from build123d import *

# Parameters (mm, degrees)
ESBO_O1_R                = 12
RESSALTO_EXTRUS_O1_DEPTH = 9.6
ESBO_O2_R                = 11.4
CORTE_EXTRUS_O1_DEPTH    = 0.1
ESBO_O3_R                = 0.5
RESSALTO_EXTRUS_O2_DEPTH = 2
ESBO_O4_R                = 1.2
CORTE_EXTRUS_O2_DEPTH    = 2
ESBO_O5_R                = 3
CORTE_EXTRUS_O3_DEPTH    = 0.3
FILETE1_R                = 1


with BuildPart() as part:
    # Esboço1 → Ressalto-extrusão1 (new body)
    with BuildSketch(Plane.XY):
        Circle(ESBO_O1_R)
    extrude(amount=RESSALTO_EXTRUS_O1_DEPTH)

    # Esboço2 → Corte-extrusão1 (cut)
    with BuildSketch(Plane(origin=(0, 0, 0), x_dir=(-1, 0, 0), z_dir=(0, 0, -1))):
        Circle(ESBO_O2_R)
    extrude(amount=-CORTE_EXTRUS_O1_DEPTH, mode=Mode.SUBTRACT)

    # Esboço3 → Ressalto-extrusão2 (add)
    with BuildSketch(Plane(origin=(0, 0, 0.1), x_dir=(-1, 0, 0), z_dir=(0, 0, -1))):
        with Locations((6, 0)):
            Circle(ESBO_O3_R)
        with Locations((-6, 0)):
            Circle(ESBO_O3_R)
    extrude(amount=RESSALTO_EXTRUS_O2_DEPTH)

    # Esboço4 → Corte-extrusão2 (cut)
    with BuildSketch(Plane.XY.offset(9.6)):
        Circle(ESBO_O4_R)
    extrude(amount=-CORTE_EXTRUS_O2_DEPTH, mode=Mode.SUBTRACT)

    # Esboço5 → Corte-extrusão3 (cut)
    with BuildSketch(Plane.XY.offset(9.6)):
        Circle(ESBO_O5_R)
    extrude(amount=-CORTE_EXTRUS_O3_DEPTH, mode=Mode.SUBTRACT)

    # Filete1
    filete1_edges = [part.edges().sort_by_distance(p)[0] for p in [
        (-12, 0, 9.6),
    ]]
    fillet(filete1_edges, radius=FILETE1_R)


solid = part.part
Geometry check sheet. Reference: the model listing, model coordinates, mm. A direction names the side the tool comes from. Give positions to 0.01 mm unless a question says otherwise; leave off trailing zeros. Loops run counter-clockwise (first coordinate to the right, second up) from the corner with the lowest first, then second, coordinate; pieces in that order, holes last. Notation, with made-up numbers: M 84,80 L 90,80 A20 cw 90,85 Z; hole C -22,-25.5 d8. An arc over 180 degrees is marked long. Answer as a JSON object with one key per item and string values. Group by question number.
Item 1: Sectioned sample at A-A on y = 0. Record the boundary of the cut face in (x, z), plus the area to 3 significant figures.
Item 2: Sectioned sample at D-D on z = 1.25. Record the boundary of the cut face in (x, y).
Item 3: Material ranges on L1, parallel to Y at x = 0, z = 8.25; L2, parallel to Z at x = -7.5, y = -2.75; L3, parallel to Y at x = 0, z = 9.5, recorded low to high.
Item 4: Mould release check, pull along Y, two halves, no side actions. Record for faces 4 (the flat face through (-6, 0, -1.9)), 5 (the cylindrical face through (-11.99, 0.53, 4.24)), 6 (the flat face through (0, 0, 7.6)): pulls with the +Y half, pulls with the -Y half, needs draft (parallel to the pull), parting line crosses it, or undercut.
Item 5: Sectioned sample at C-C on z = -0.5. Record the boundary of the cut face in (x, y).
Item 6: Access from +Z, -Z, +X, -X, +Y, -Y to the whole of each face (thin tool, end or side, straight path). Record for faces 1 (the flat face through (1, -1, 9.3)), 2 (the flat face through (0, 0, 0.1)), 3 (the flat face through (2.3, -2.3, 9.6)).
Item 7: Gauge pin test, flat ends, axial feed: pin 1 (3 mm diameter, centred on x = 0, y = 0, fed in from -Z); pin 2 (2.5 mm diameter, centred on x = 0, y = 0, fed in from +Z); pin 3 (1.5 mm diameter, centred on y = 1, z = 4, fed in from +X); pin 4 (11.5 mm diameter, centred on x = 4.5, y = -1.5, fed in from -Z). Record the tip position at first contact, or that the pin passes through.
Item 8: Sectioned sample at B-B on x = 0. Record the boundary of the cut face in (y, z).
Findings below:
{
 "1": {"outline": "M -12,0 L -11.4,0 L -11.4,0.1 L -6.5,0.1 L -6.5,-1.9 L -5.5,-1.9 L -5.5,0.1 L 5.5,0.1 L 5.5,-1.9 L 6.5,-1.9 L 6.5,0.1 L 11.4,0.1 L 11.4,0 L 12,0 L 12,8.6 A1 ccw 11,9.6 L 3,9.6 L 3,9.3 L 1.2,9.3 L 1.2,7.6 L -1.2,7.6 L -1.2,9.3 L -3,9.3 L -3,9.6 L -11,9.6 A1 ccw -12,8.6 Z", "area": "226 mm2"},
 "2": {"outline": "C 0,0 d24"},
 "3": {"L1": "-12 to -1.2, 1.2 to 12", "L2": "0.1 to 9.6", "L3": "-11.44 to -3, 3 to 11.44"},
 "4": {"face 4": "needs draft", "face 5": "parting line crosses it", "face 6": "undercut"},
 "5": {"outline": "C -6,0 d1; C 6,0 d1"},
 "6": {"face 1": "+Z", "face 2": "-Z", "face 3": "+Z, +X, -X, +Y, -Y"},
 "7": {"pin 1": "z = 0.1", "pin 2": "z = 9.3", "pin 3": "x = 12", "pin 4": "z = -1.9"},
 "8": {"outline": "M -12,0 L -11.4,0 L -11.4,0.1 L 11.4,0.1 L 11.4,0 L 12,0 L 12,8.6 A1 ccw 11,9.6 L 3,9.6 L 3,9.3 L 1.2,9.3 L 1.2,7.6 L -1.2,7.6 L -1.2,9.3 L -3,9.3 L -3,9.6 L -11,9.6 A1 ccw -12,8.6 Z"}
}
